Part model, mm, in its own coordinate system. Coordinates: 2 decimals unless noted, no trailing zeros. Loops run counter-clockwise (first coordinate to the right, second up) from the corner with the lowest first, then second, coordinate; pieces in that order, holes last.
```python
from build123d import *

# Parameters (mm, degrees)
SKETCH1_W           = 37
SKETCH1_H           = 37
BOSS_EXTRUDE1_DEPTH = 899
CUT_EXTRUDE2_DEPTH  = 20
SKETCH4_W           = 8
SKETCH4_H           = 41
CUT_EXTRUDE3_DEPTH  = 901.777997067
SKETCH5_R           = 3.58636949
CUT_EXTRUDE4_DEPTH  = 10
CUT_EXTRUDE5_DEPTH  = 20
SKETCH7_R           = 3
CUT_EXTRUDE6_DEPTH  = 901.777997067


with BuildPart() as part:
    # Sketch1 → Boss-Extrude1 (new body)
    with BuildSketch(Plane(origin=(0, 0, 0), x_dir=(1, 0, 0), z_dir=(0, 1, 0))):
        with BuildLine():
            Line((0.5, 0), (39.5, 0))
            ThreePointArc((39.5, 0), (39.853553391, 0.146446609), (40, 0.5))
            Line((40, 0.5), (40, 39.5))
            ThreePointArc((40, 39.5), (39.853553391, 39.853553391), (39.5, 40))
            Line((39.5, 40), (0.5, 40))
            ThreePointArc((0.5, 40), (0.146446609, 39.853553391), (0, 39.5))
            Line((0, 39.5), (0, 0.5))
            ThreePointArc((0, 0.5), (0.146446609, 0.146446609), (0.5, 0))
        make_face()
        with Locations((20, 20)):
            Rectangle(SKETCH1_W, SKETCH1_H, mode=Mode.SUBTRACT)
    extrude(amount=BOSS_EXTRUDE1_DEPTH)

    # Sketch3 → Cut-Extrude2 (cut)
    with BuildSketch(Plane.XY):
        Polygon((40, 5.907288086), (37, 5.907288086), (37, 7.639845548), (22.874509033, 15.797587142), (32.926772366, 32.098076211), (37, 29.74639714), (40, 29.74639714), (40, 28.014346333), align=None)
    extrude(amount=-CUT_EXTRUDE2_DEPTH, mode=Mode.SUBTRACT)

    # Sketch4 → Cut-Extrude3 (cut, through all)
    with BuildSketch(Plane.ZY):
        with Locations((-4, 878.5)):
            Rectangle(SKETCH4_W, SKETCH4_H)
        with Locations((-36, 878.5)):
            Rectangle(SKETCH4_W, SKETCH4_H)
    extrude(amount=-CUT_EXTRUDE3_DEPTH, mode=Mode.SUBTRACT)

    # Sketch5 → Cut-Extrude4 (cut)
    with BuildSketch(Plane(origin=(0, 0, -40), x_dir=(-1, 0, 0), z_dir=(0, 0, -1))):
        with Locations((-30, 30)):
            Circle(SKETCH5_R)
        with Locations((-30, 15)):
            Circle(SKETCH5_R)
    extrude(amount=-CUT_EXTRUDE4_DEPTH, mode=Mode.SUBTRACT)

    # Sketch6 → Cut-Extrude5 (cut)
    with BuildSketch(Plane(origin=(40, 0, 0), x_dir=(0, 0, -1), z_dir=(1, 0, 0))):
        Polygon((0, 708.5), (20, 708.5), (20, 668), (10, 668), (10, 688), (0, 688), align=None)
        Polygon((0, 518.5), (20, 518.5), (20, 478), (10, 478), (10, 498), (0, 498), align=None)
        Polygon((0, 328.5), (20, 328.5), (20, 288), (10, 288), (10, 308), (0, 308), align=None)
        Polygon((0, 138.5), (20, 138.5), (20, 98), (10, 98), (10, 118), (0, 118), align=None)
    extrude(amount=-CUT_EXTRUDE5_DEPTH, mode=Mode.SUBTRACT)

    # Sketch7 → Cut-Extrude6 (cut, through all)
    with BuildSketch(Plane.XY):
        with Locations((20, 84)):
            Circle(SKETCH7_R)
    extrude(amount=-CUT_EXTRUDE6_DEPTH, mode=Mode.SUBTRACT)


solid = part.part
```
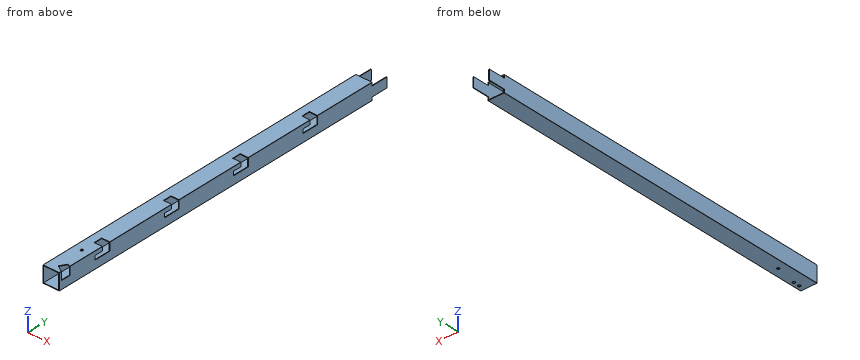
Q1. Probe line 1 (Y direction, x = 30, z = -39.05); line 2 (Z direction, x = 25.5, y = 571); line 3 (X direction, y = 698.5, z = -20.5). List the from-to ranges inside material, lowest first.
Q2. Saw through at C-C (y = 320). List the corners of the cut face in (x, z).
Q3. Drop flat-ended pins along their axis: P1, Ø0.8, axis at x = 39.5, y = 877.5, coming from the +Z side; P2, Ø8, axis at x = 30, y = 15, coming from the +Z side; P3, Ø6.5, axis at x = 30, y = 30, coming from the -Z side; P4, Ø1.6, axis at x = 0.5, y = 882.5, coming from the -Z side. Give the stop position or say it passes through.
Q4. Saw through at A-A (x = 8.5). List the corners of the cut face in (y, z).
Q5. Saw through at B-B (y = 629). List the corners of the cut face in (x, z), plus the area to 3 significant figures.
Checked values:
1. line 1: y = 0 to 11.41, 18.59 to 26.41, 33.59 to 858
1. line 2: z = -40 to -38.5, -1.5 to 0
1. line 3: x = 0 to 1.5, 38.5 to 40
2. outline: (0, -39.5) arc R0.5 ccw to (0.5, -40) - (39.5, -40) arc R0.5 ccw to (40, -39.5) - (40, -20) - (38.5, -20) - (38.5, -38.5) - (1.5, -38.5) - (1.5, -1.5) - (20, -1.5) - (20, 0) - (0.5, 0) arc R0.5 ccw to (0, -0.5) - close
3. P1: stops at z = -8
3. P2: stops at z = 0
3. P3: stops at z = -1.5
3. P4: stops at z = -32
4. outline: (0, -40) - (858, -40) - (858, -38.5) - (0, -38.5) - close; (0, -1.5) - (858, -1.5) - (858, 0) - (0, 0) - close
5. outline: (0, -39.5) arc R0.5 ccw to (0.5, -40) - (39.5, -40) arc R0.5 ccw to (40, -39.5) - (40, -0.5) arc R0.5 ccw to (39.5, 0) - (0.5, 0) arc R0.5 ccw to (0, -0.5) - close; hole (1.5, -38.5) - (38.5, -38.5) - (38.5, -1.5) - (1.5, -1.5) - close
5. area: 231 mm2
